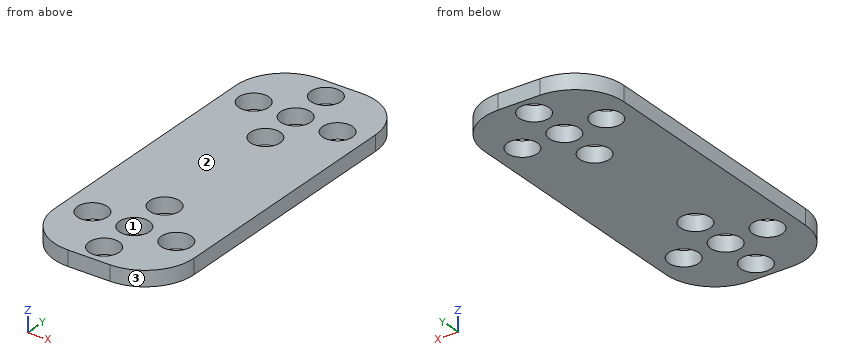
Autodesk Inventor part; units mm, degrees
ref_plane "YZ Plane" through (0, 0, 0) normal (1, 0, 0) x (0, 1, 0)
ref_plane "XZ Plane" through (0, 0, 0) normal (0, 1, 0) x (-1, 0, 0)
ref_plane "XY Plane" through (0, 0, 0) normal (0, 0, 1) x (1, 0, 0)
sketch "Esquisse5" plane through (0, 0, 0) normal (0, 0, 1) x (1, 0, 0)
  line L0 (0, 0) -> (20, 0)
  line L1 (20, 0) -> (20, 25)
  line L2 (20, 25) -> (0, 25)
  line L3 (0, 25) -> (0, 0)
  line L4 (10, 0) -> (10, 25) construction
  circle A0 centre (10, 3) radius 2.15
  circle A1 centre (10, 9) radius 2.15
  circle A2 centre (10, 15) radius 2.15
  line L5 (10, 9) -> (20, 9) construction
  circle A3 centre (16, 9) radius 2.15
  circle A4 centre (4, 9) radius 2.15
  circle A5 centre (10, 9) radius 2.15
  dimension "d61" = 20
  dimension "d62" = 25
  dimension "d63" = 3
  dimension "d64" = 4.3
  dimension "d67" = 6
  dimension "d74" = 6
  dimension "d77" = 6
extrude "Extrusion5" add sketch "Esquisse5" along normal blind 2.2
fillet "Congé4" radius 7 2 edges at (0, 0, 1.1) (20, 0, 1.1)
mirror "Symétrie1" about plane through (20, 25, 0) normal (0, 1, 0)
equation "\"d64\" = Holes"
equation "\"d80\" = Depth"
equation "\"d100\" = Rounding"
equation "\"Depth\" = 2.2"
equation "\"Holes\" = 4.3"
equation "\"Height\" = 0"
equation "\"Rounding\" = 7"
properties part number "ArmToArm"
Read the model definition and answer for the solid it produces. Units are mm, in the model's axes. Face numbers are marked on the shaded views. Coordinates: 2 decimals unless noted, no trailing zeros. Write each loop counter-clockwise with the first axis right and the second up, starting at its lowest first coordinate (ties: lowest second). Pieces come first, ordered by that corner, then holes. Notation, with made-up numbers: M -25,-34 L 19,-34 A8 cw 19,-22 Z; hole C -14,-34.5 d5. An arc over 180 degrees is marked long. Use a Markdown table: item, result.
Q1. The part is cut by section B-B, the plane z = 0.85. Give the number of separate pieces and of enclosed holes in the cut face, then the cut area to 3 significant figures.
Answer block:
| item | result |
|---|---|
| separate pieces | 1 |
| enclosed holes | 10 |
| area | 813 mm2 |
Q2. Straight lines are drawn through the part: L1, parallel to X at y = 41, z = 1.7; L2, parallel to X at y = 10, z = 0.5; L3, parallel to Y at x = 2.25, z = 1.5. For each, find the intervals that lie inside material, in ascending order. Write a range as [from, to].
Answer block:
| item | result |
|---|---|
| L1 | x = [0, 1.85], [6.15, 7.85], [12.15, 13.85], [18.15, 20] |
| L2 | x = [0, 2.1], [5.9, 8.1], [11.9, 14.1], [17.9, 20] |
| L3 | y = [1.86, 7.75], [10.25, 39.75], [42.25, 48.14] |
Q3. Determine the mould class of the marked faces 1, 2 and 3 for opening direction Y: released by +Y, released by -Y, zero draft, split by the parting line, or undercut.
Answer block:
| item | result |
|---|---|
| face 1 | undercut |
| face 2 | zero draft |
| face 3 | released by -Y |
Q4. The part is cut by section C-C, the plane y = 35. Write down the section's boundary in (x, z).
Answer block:
| item | result |
|---|---|
| outline | M 0,0 L 7.85,0 L 7.85,2.2 L 0,2.2 Z; M 12.15,0 L 20,0 L 20,2.2 L 12.15,2.2 Z |
Q5. This flat-tipped pin is pushed along its axis until it touches: pin 1 Ø3.5 at (x, y) = (16, 41) entering from +Z. Where does it stop, or does it pass through?
Answer block:
| item | result |
|---|---|
| pin 1 | passes through |
Q6. The part is cut by section D-D, the plane x = 4. Write down the section's boundary in (y, z), then the cut area to 3 significant figures.
Answer block:
| item | result |
|---|---|
| outline | M 0.68,0 L 6.85,0 L 6.85,2.2 L 0.68,2.2 Z; M 11.15,0 L 38.85,0 L 38.85,2.2 L 11.15,2.2 Z; M 43.15,0 L 49.32,0 L 49.32,2.2 L 43.15,2.2 Z |
| area | 88.1 mm2 |
Q7. The part is cut by section A-A, the plane y = 41. Write down the section's boundary in (x, z).
Answer block:
| item | result |
|---|---|
| outline | M 0,0 L 1.85,0 L 1.85,2.2 L 0,2.2 Z; M 6.15,0 L 7.85,0 L 7.85,2.2 L 6.15,2.2 Z; M 12.15,0 L 13.85,0 L 13.85,2.2 L 12.15,2.2 Z; M 18.15,0 L 20,0 L 20,2.2 L 18.15,2.2 Z |
